```python
from build123d import *

# Parameters (mm, degrees)
F2_W     = 30
F2_H     = 60
F3_DEPTH = 5
F4_W     = 30
F4_H     = 15
F5_DEPTH = 55
F6_W     = 20
F6_H     = 5
F7_DEPTH = 47.501


with BuildPart() as f3:
    # F2 (on Top) → F3 (new body)
    with BuildSketch(Plane.XY):
        with Locations((0, 10)):
            Rectangle(F2_W, F2_H)
    extrude(amount=F3_DEPTH)

    # F4 (on face) → F5 (join)
    with BuildSketch(Plane.XY.offset(5)):
        Rectangle(F4_W, F4_H)
    extrude(amount=F5_DEPTH)

    # F6 (on face) → F7 (cut, through all)
    with BuildSketch(Plane.XZ.offset(7.5)):
        with Locations((0, 51)):
            Rectangle(F6_W, F6_H)
        with Locations((0, 33)):
            Rectangle(F6_W, F6_H)
        with Locations((0, 18)):
            Rectangle(F6_W, F6_H)
    extrude(amount=-F7_DEPTH, mode=Mode.SUBTRACT)


solid = f3.part
```
Geometry: final body of the model. Coordinates: model frame, mm. A direction names the side the tool comes from. Round coordinates to 2 decimals unless told otherwise and drop trailing zeros. Loops run counter-clockwise (first coordinate to the right, second up) from the corner with the lowest first, then second, coordinate; pieces in that order, holes last. Notation, with made-up numbers: (-14.5, 73.5) -> (15.5, 73.5) arc R9 ccw to (15.5, 83.5) -> close; hole circle Ø10 at (-9, 10.25). An arc over 180 degrees is marked (long way). Use one line per item in the form item = value.
Item 1: Draft query along X for faces 4 (the flat face through (15, 3, 23)), 5 (the flat face through (0, 0, 53.5)), 6 (the flat face through (0, -14, 5)). Return one class per face: released by +X, released by -X, zero draft, split by the parting line, or undercut.
Evaluation:
face_4 = released by +X
face_5 = undercut
face_6 = zero draft
Item 2: Cut plane D-D on y = 25. Output: boundary loops of the cut face in (x, z).
Evaluation:
outline = (-15, 0) -> (15, 0) -> (15, 5) -> (-15, 5) -> close
Item 3: Contact query for flat-ended pins moving along their axis: pin 1 Ø6 at (x, y) = (2, 18) entering from +Z; pin 2 Ø2 at (x, z) = (6.5, 24.5) entering from -Y. Output: stop coordinate, or through.
Evaluation:
pin_1 = 5
pin_2 = -7.5
Item 4: Cut plane A-A on x = 2. Output: boundary loops of the cut face in (y, z).
Evaluation:
outline = (-20, 0) -> (40, 0) -> (40, 5) -> (7.5, 5) -> (7.5, 15.5) -> (-7.5, 15.5) -> (-7.5, 5) -> (-20, 5) -> close; (-7.5, 20.5) -> (7.5, 20.5) -> (7.5, 30.5) -> (-7.5, 30.5) -> close; (-7.5, 35.5) -> (7.5, 35.5) -> (7.5, 48.5) -> (-7.5, 48.5) -> close; (-7.5, 53.5) -> (7.5, 53.5) -> (7.5, 60) -> (-7.5, 60) -> close
Item 5: Access query for faces 1 (the flat face through (0, -7.5, 26)), 2 (the flat face through (0, 24, 5)), 3 (the flat face through (0, 0, 15.5)). Directions: +Z, -Z, +X, -X, +Y, -Y. A direction counts if a zero-diameter tool reaches every point of the face in a straight line with its end or side. Return the directions, or none.
Evaluation:
face_1 = +Z, +X, -X, -Y
face_2 = +Z, +X, -X, +Y
face_3 = +Y, -Y
Item 6: Cut plane B-B on y = -3.5. Output: boundary loops of the cut face in (x, z).
Evaluation:
outline = (-15, 0) -> (15, 0) -> (15, 60) -> (-15, 60) -> close; hole (-10, 15.5) -> (10, 15.5) -> (10, 20.5) -> (-10, 20.5) -> close; hole (-10, 30.5) -> (10, 30.5) -> (10, 35.5) -> (-10, 35.5) -> close; hole (-10, 48.5) -> (10, 48.5) -> (10, 53.5) -> (-10, 53.5) -> close
Item 7: Cut plane C-C on x = -12.75. Output: boundary loops of the cut face in (y, z).
Evaluation:
outline = (-20, 0) -> (40, 0) -> (40, 5) -> (7.5, 5) -> (7.5, 60) -> (-7.5, 60) -> (-7.5, 5) -> (-20, 5) -> close
Item 8: Material intervals for probe 1 along Z at (x, y) = (-5.5, -5); probe 2 along X at (y, z) = (0, 19); probe 3 along Y at (x, z) = (7.75, 37), sorted ascending.
Evaluation:
probe_1 = 0 to 15.5, 20.5 to 30.5, 35.5 to 48.5, 53.5 to 60
probe_2 = -15 to -10, 10 to 15
probe_3 = -7.5 to 7.5
